Check sheet for the modelled part. Datum: model origin and axes. Units: mm. A direction names the side the tool comes from. Give positions to 0.01 mm unless a question says otherwise; leave off trailing zeros. Loops run counter-clockwise (first coordinate to the right, second up) from the corner with the lowest first, then second, coordinate; pieces in that order, holes last. Notation, with made-up numbers: M 43,69 L 51,69 A30 ccw 51,93 Z; hole C 51.5,81.5 d1. An arc over 180 degrees is marked long. One line per question, with ' | ' between items. Start each with the question number.
from build123d import *

# Parameters (mm, degrees)
SKETCH1_R           = 24.75
BOSS_EXTRUDE1_DEPTH = 58.2
SKETCH2_R           = 4
BOSS_EXTRUDE2_DEPTH = 22.5
CHAMFER1_SIZE       = 2.5
SKETCH3_R           = 6.8
BOSS_EXTRUDE3_DEPTH = 2
FILLET1_R           = 0.5
SKETCH4_R           = 2
CUT_EXTRUDE1_DEPTH  = 10
SKETCH5_R           = 1.5
CUT_EXTRUDE2_DEPTH  = 5
CHAMFER2_SIZE       = 9.5
CHAMFER2_SIZE2      = 2
CUT_EXTRUDE3_DEPTH  = 8.5
SKETCH7_W           = 12.5
SKETCH7_H           = 5.5
CUT_EXTRUDE4_DEPTH  = 8.5


with BuildPart() as part:
    # Sketch1 → Boss-Extrude1 (new body)
    with BuildSketch(Plane(origin=(0, 0, 0), x_dir=(1, 0, 0), z_dir=(0, 1, 0))):
        with Locations(Location((0, 0, 0), (0, 0, 270))):
            Circle(SKETCH1_R)
    extrude(amount=BOSS_EXTRUDE1_DEPTH)

    # Sketch2 → Boss-Extrude2 (add)
    with BuildSketch(Plane(origin=(0, 58.2, 0), x_dir=(1, 0, 0), z_dir=(0, 1, 0))):
        with Locations(Location((0, 0, 0), (0, 0, 90))):
            Circle(SKETCH2_R)
    extrude(amount=BOSS_EXTRUDE2_DEPTH)

    # Chamfer1
    chamfer1_edges = [part.edges().sort_by_distance(p)[0] for p in [
        (0, 0, -24.75),
    ]]
    chamfer(chamfer1_edges, length=CHAMFER1_SIZE)

    # Sketch3 → Boss-Extrude3 (add)
    with BuildSketch(Plane.XZ):
        with Locations(Location((0, 0, 0), (0, 0, 270))):
            Circle(SKETCH3_R)
    extrude(amount=BOSS_EXTRUDE3_DEPTH)

    # Fillet1
    fillet1_edges = [part.edges().sort_by_distance(p)[0] for p in [
        (0, 0, 6.8),
    ]]
    fillet(fillet1_edges, radius=FILLET1_R)

    # Sketch4 → Cut-Extrude1 (cut)
    with BuildSketch(Plane(origin=(0, 58.2, 0), x_dir=(1, 0, 0), z_dir=(0, 1, 0))):
        with Locations(Location((0, 15, 0), (0, 0, 270))):
            Circle(SKETCH4_R)
        with Locations(Location((15, 0, 0), (0, 0, 270))):
            Circle(SKETCH4_R)
        with Locations(Location((0, -15, 0), (0, 0, 270))):
            Circle(SKETCH4_R)
        with Locations(Location((-15, 0, 0), (0, 0, 270))):
            Circle(SKETCH4_R)
    extrude(amount=-CUT_EXTRUDE1_DEPTH, mode=Mode.SUBTRACT)

    # Sketch5 → Cut-Extrude2 (cut)
    with BuildSketch(Plane.XZ):
        with Locations(Location((0, 9.875, 0), (0, 0, 270))):
            Circle(SKETCH5_R)
        with Locations(Location((9.875, 0, 0), (0, 0, 270))):
            Circle(SKETCH5_R)
        with Locations(Location((0, -9.875, 0), (0, 0, 270))):
            Circle(SKETCH5_R)
        with Locations(Location((-9.875, 0, 0), (0, 0, 270))):
            Circle(SKETCH5_R)
    extrude(amount=-CUT_EXTRUDE2_DEPTH, mode=Mode.SUBTRACT)

    # Chamfer2
    chamfer2_edges = [part.edges().sort_by_distance(p)[0] for p in [
        (0, 58.2, -24.75),
    ]]
    chamfer2_side = [part.faces().sort_by_distance(p)[0] for p in [
        (0, 30.35, -24.75),
    ]]
    chamfer(chamfer2_edges, length=CHAMFER2_SIZE, length2=CHAMFER2_SIZE2, reference=chamfer2_side[0])

    # Sketch6 → Cut-Extrude3 (cut)
    with BuildSketch(Plane(origin=(0, 58.2, 0), x_dir=(1, 0, 0), z_dir=(0, 1, 0))):
        Polygon((19.516147161, -10.677312396), (10.677312396, -19.516147161), (17.748380208, -26.587214973), (26.587214973, -17.748380208), align=None)
    extrude(amount=-CUT_EXTRUDE3_DEPTH, mode=Mode.SUBTRACT)

    # Sketch7 → Cut-Extrude4 (cut)
    with BuildSketch(Plane(origin=(15.096729778, 0, 15.096729778), x_dir=(0.7071067811865476, 0, -0.7071067811865476), z_dir=(0.7071067811865476, 0, 0.7071067811865476))):
        with Locations((0, 52.45)):
            Rectangle(SKETCH7_W, SKETCH7_H)
    extrude(amount=-CUT_EXTRUDE4_DEPTH, mode=Mode.SUBTRACT)


solid = part.part
Q1. Cross-section at D-D (y = 14). Record the cut outline in (x, z), and give its area (3 significant figures).
Q2. Material ranges on probe 1 along X at (y, z) = (52.75, 0); probe 2 along Y at (x, z) = (-2, 9); probe 3 along Y at (x, z) = (16, 11), recorded low to high. Write a range as from..to.
Q3. Draft check along Z on faces 5 (the cylindrical face through (3.905, 69.292, 0.867)), 6 (the flat face through (0, 80.7, 0)), 7 (the cylindrical face through (-1.2, 53.3, 13.4)). Enter one of: released by +Z, released by -Z, zero draft, split by the parting line, or undercut.
Q4. Depth check by flat-ended pin: P1, Ø8, axis at x = 7.5, y = 34, coming from the -Z side; P2, Ø6, axis at x = 0, z = -12, coming from the +Y side; P3, Ø3, axis at x = 3.5, z = -14, coming from the -Y side. Enter the tip coordinate at first touch or a pass-through.
Q5. Cross-section at B-B (y = 3.5). Record the cut outline in (x, z) (3 decimals), and give its area (3 significant figures).
Q6. Access from +Z, -Z, +X, -X, +Y, -Y to the whole of each face (thin tool, end or side, straight path). Record for faces 1 (the flat face through (13, 49.7, 13)), 2 (the cylindrical face through (16.73, 25.28, -18.24)), 3 (the flat face through (-10, 5, 0)), 4 (the flat face through (15, 48.2, 0)).
Solved:
1) outline: C 0,0 d49.5 | area: 1,920 mm²
2) probe 1: x = -23.9..-17, -13..13, 17..23.9 | probe 2: y = 0..58.2 | probe 3: y = 0..49.7, 55.2..58.2
3) face 5: split by the parting line | face 6: zero draft | face 7: undercut
4) P1: stops at z = -24.5 | P2: stops at y = 58.2 | P3: stops at y = 0
5) outline: C 0,0 d49.5; hole C -9.875,0 d3; hole C 0,-9.875 d3; hole C 0,9.875 d3; hole C 9.875,0 d3 | area: 1,900 mm²
6) face 1: none | face 2: +Y, -Y | face 3: -Y | face 4: +Y
